from build123d import *

# Parameters (mm, degrees)
SKETCH1_W                        = 50.8
SKETCH1_H                        = 101.6
EXTRUDE1_DEPTH                   = 152.4
SKETCH2_R                        = 22.225
EXTRUDE2_DEPTH                   = 51.8
CHAMFER1_SIZE                    = 2.54
F_3_8_16_TAPPED_HOLE1_AT_2_COUNT = 2
F_3_8_16_TAPPED_HOLE1_AT_2_PITCH = 50.8


with BuildPart() as part:
    # Sketch1 → Extrude1 (new body)
    with BuildSketch(Plane.XY):
        with Locations((25.4, 0)):
            Rectangle(SKETCH1_W, SKETCH1_H)
    extrude(amount=EXTRUDE1_DEPTH)

    # Sketch2 → Extrude2 (cut, through all)
    with BuildSketch(Plane(origin=(50.8, 0, 0), x_dir=(0, 0, -1), z_dir=(1, 0, 0))):
        with Locations(Location((-114.3, 0, 0), (0, 0, 90))):  # turned: the seam where the file's is
            Circle(SKETCH2_R)
    extrude(amount=-EXTRUDE2_DEPTH, mode=Mode.SUBTRACT)

    # Chamfer1
    chamfer1_edges = [part.edges().sort_by_distance(p)[0] for p in [
        (50.8, -22.225, 114.3),
        (50.8, -50.8, 76.2),
        (0, -50.8, 76.2),
        (0, 50.8, 76.2),
        (50.8, 50.8, 76.2),
    ]]
    chamfer(chamfer1_edges, length=CHAMFER1_SIZE)

    # Sketch3 → 3/8-16 Tapped Hole1 (revolve, cut)
    with BuildSketch(Plane(origin=(25.4, -25.4, 0), x_dir=(0, 1, 0), z_dir=(1, 0, 0))):
        Polygon((0, 0), (0, 26.260665582), (3.96875, 23.876), (3.96875, 1.42875), (5.3975, 0), align=None)
    f_3_8_16_tapped_hole1 = revolve(axis=Axis((25.4, -25.4, -6.35), (0, 0, 1)), mode=Mode.SUBTRACT)

    # 3/8-16 Tapped Hole1 at 2: 3/8-16 Tapped Hole1 ×2
    with Locations(*[(0, i * F_3_8_16_TAPPED_HOLE1_AT_2_PITCH, 0) for i in range(1, F_3_8_16_TAPPED_HOLE1_AT_2_COUNT)]):
        add(f_3_8_16_tapped_hole1, mode=Mode.SUBTRACT)

    # Mirror1: 3/8-16 Tapped Hole1 across plane
    add(f_3_8_16_tapped_hole1.mirror(Plane(origin=(0, 0, 76.2), x_dir=(1, 0, 0), z_dir=(0, 0, -1))), mode=Mode.SUBTRACT)

    # Mirror1 copy 1 sketch → Mirror1 copy 1 (revolve, cut)
    with BuildSketch(Plane(origin=(25.4, 25.4, 152.4), x_dir=(0, 1, 0), z_dir=(1, 0, 0))):
        Polygon((0, 0), (0, -26.260665582), (3.96875, -23.876), (3.96875, -1.42875), (5.3975, 0), align=None)
    revolve(axis=Axis((25.4, 25.4, 158.75), (0, 0, 1)), mode=Mode.SUBTRACT)


solid = part.part
Geometry check sheet. Reference: the model listing, model coordinates, mm. A direction names the side the tool comes from. Give positions to 0.01 mm unless a question says otherwise; leave off trailing zeros. Order: outer loops, then holes, each group sorted by start corner. A loop starts at its lowest first (then second) coordinate and runs counter-clockwise, first axis right, second up.
1. Scan lines: line 1 (Y direction, x = 25.4, z = 145.25); line 2 (Y direction, x = 33, z = 114); line 3 (Y direction, x = 25, z = 18). Record each from-to range of solid material in increasing order.
Completed:
line 1: y = -50.8 to -29.37, -21.43 to 21.43, 29.37 to 50.8
line 2: y = -50.8 to -22.22, 22.22 to 50.8
line 3: y = -50.8 to -29.35, -21.45 to 21.45, 29.35 to 50.8
2. Depth check by flat-ended pin: pin 1 (12.5 mm diameter, centred on x = 25.4, y = -25.4, fed in from -Z); pin 2 (9 mm diameter, centred on x = 25.4, y = 25.4, fed in from -Z); pin 3 (6.5 mm diameter, centred on x = 25.4, y = 25.4, fed in from +Z). Enter the tip coordinate at first touch or a pass-through.
Completed:
pin 1: stops at z = 0
pin 2: stops at z = 0.9
pin 3: stops at z = 128.09
3. Access from +Z, -Z, +X, -X, +Y, -Y to the whole of each face (thin tool, end or side, straight path). Record for faces 4 (the face through (27.815, 22.251, 139.905)), 5 (the face through (24.5, -16.4, 129.3)), 6 (the face through (27.815, 22.251, 12.495)).
Completed:
face 4: +Z
face 5: +X, -X
face 6: -Z
4. Draft check along X on faces 1 (the face through (48.419, -2.914, 136.493)), 2 (the face through (27.815, -28.549, 12.495)), 3 (the face through (25, 1, 152.4)). Enter one of: pulls with the +X half, pulls with the -X half, needs draft (parallel to the pull), parting line crosses it, or undercut.
Completed:
face 1: pulls with the +X half
face 2: undercut
face 3: needs draft
5. Sectioned sample at B-B (x = 44). Record the boundary of the cut face in (y, z) (3 decimals).
Completed:
outline: (-50.8, 0) - (50.8, 0) - (50.8, 152.4) - (-50.8, 152.4) - close; hole circle Ø44.45 at (0, 114.3)
6. Sectioned sample at A-A (y = 0). Record the boundary of the cut face in (x, z) (3 decimals), then the cut area to 3 significant figures.
Completed:
outline: (0, 0) - (50.8, 0) - (50.8, 89.535) - (48.26, 92.075) - (0, 92.075) - close; (0, 136.525) - (48.26, 136.525) - (50.8, 139.065) - (50.8, 152.4) - (0, 152.4) - close
area: 5,480 mm2
